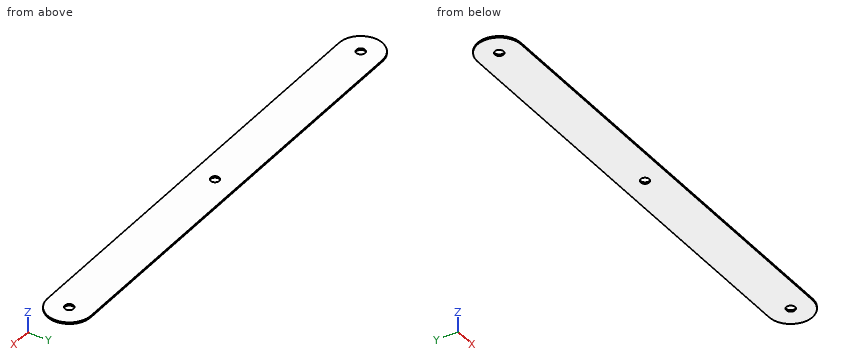
from build123d import *

# Parameters (mm, degrees)
SKETCH1_R          = 2
BASE_FLANGE1_DEPTH = 0.7366


# Sheet-metal steps are written as plain solids
with BuildPart() as part:
    # Sketch1 → Base-Flange1 (new body)
    with BuildSketch(Plane.XY):
        with BuildLine():
            Line((-28.344481605, 10), (171.655518395, 10))
            ThreePointArc((171.655518395, 10), (181.655518395, 0), (171.655518395, -10))
            Line((171.655518395, -10), (-28.344481605, -10))
            ThreePointArc((-28.344481605, -10), (-38.344481605, 0), (-28.344481605, 10))
        make_face()
        with Locations((-28.344481605, 0)):
            Circle(SKETCH1_R, mode=Mode.SUBTRACT)
        with Locations((171.655518395, 0)):
            Circle(SKETCH1_R, mode=Mode.SUBTRACT)
        with Locations((71.655518395, 0)):
            Circle(SKETCH1_R, mode=Mode.SUBTRACT)
    extrude(amount=-BASE_FLANGE1_DEPTH)


solid = part.part
Read the model definition and answer for the solid it produces. Units are mm, in the model's axes. Round coordinates to 2 decimals unless told otherwise and drop trailing zeros. Write each loop counter-clockwise with the first axis right and the second up, starting at its lowest first coordinate (ties: lowest second). Pieces come first, ordered by that corner, then holes.
1. The part is cut by section A-A, the plane z = -0.25. Determine the outline of the cut face in (x, y), then the cut area to 3 significant figures.
2. Given pin 1 Ø3 at (x, y) = (171.66, 0) entering from +Z, flat-ended and moving along its own axis, determine where the tip first touches the part or whether it passes through.
3. Straight lines are drawn through the part: L1, parallel to X at y = 1.25, z = -0.5; L2, parallel to X at y = -4.75, z = -0.55; L3, parallel to X at y = -3.5, z = -0.3. For each, find the intervals that lie inside material, in ascending order.
4. The part is cut by section B-B, the plane y = 0. Determine the outline of the cut face in (x, z).
5. The part is cut by section C-C, the plane y = -8. Determine the outline of the cut face in (x, z).
Values:
1. outline: (-28.34, -10) - (171.66, -10) arc R10 ccw to (171.66, 10) - (-28.34, 10) arc R10 ccw to start; hole circle Ø4 at (-28.34, 0); hole circle Ø4 at (71.66, 0); hole circle Ø4 at (171.66, 0)
1. area: 4,280 mm2
2. pin 1: passes through
3. L1: x = -38.27 to -29.91, -26.78 to 70.09, 73.22 to 170.09, 173.22 to 181.58
3. L2: x = -37.14 to 180.46
3. L3: x = -37.71 to 181.02
4. outline: (-38.34, -0.74) - (-30.34, -0.74) - (-30.34, 0) - (-38.34, 0) - close; (-26.34, -0.74) - (69.66, -0.74) - (69.66, 0) - (-26.34, 0) - close; (73.66, -0.74) - (169.66, -0.74) - (169.66, 0) - (73.66, 0) - close; (173.66, -0.74) - (181.66, -0.74) - (181.66, 0) - (173.66, 0) - close
5. outline: (-34.34, -0.74) - (177.66, -0.74) - (177.66, 0) - (-34.34, 0) - close
